Geometry: final body of the model. Coordinates: model frame, mm. A direction names the side the tool comes from. Coordinates: 2 decimals unless noted, no trailing zeros. Order: outer loops, then holes, each group sorted by start corner. A loop starts at its lowest first (then second) coordinate and runs counter-clockwise, first axis right, second up. Notation, with made-up numbers: (54, -20) - (72, -20) arc R12 cw to (72, -9) - close; hole circle Ø10 at (-21, 9). An arc over 180 degrees is marked (long way). Use one line per item in the form item = value. Start each with the question number.
```python
from build123d import *

# Parameters (mm, degrees)
SKETCH1_R               = 38.1
BOSS_EXTRUDE1_DEPTH     = 12.7
SKETCH2_W               = 30.48
SKETCH2_H               = 50.8
BOSS_EXTRUDE2_DEPTH     = 10.16
SKETCH3_W               = 25.4
SKETCH3_H               = 45.72
CUT_EXTRUDE1_DEPTH      = 10.16
BOSS_EXTRUDE3_DEPTH     = 127
SKETCH5_R               = 1.27
CUT_EXTRUDE2_DEPTH      = 5.08
SKETCH6_R               = 5.08
CUT_EXTRUDE3_DEPTH      = 5.08
SKETCH7_R               = 1.905
CUT_EXTRUDE4_DEPTH      = 57.658
CUT_EXTRUDE4_DEPTH_BACK = 54.61


with BuildPart() as part:
    # Sketch1 → Boss-Extrude1 (new body)
    with BuildSketch(Plane(origin=(0, 0, 0), x_dir=(1, 0, 0), z_dir=(0, 1, 0))):
        with Locations(Location((0, 0, 0), (0, 0, 270))):
            Circle(SKETCH1_R)
    extrude(amount=BOSS_EXTRUDE1_DEPTH)

    # Sketch2 → Boss-Extrude2 (add)
    with BuildSketch(Plane(origin=(0, 12.7, 0), x_dir=(1, 0, 0), z_dir=(0, 1, 0))):
        Rectangle(SKETCH2_W, SKETCH2_H)
    extrude(amount=BOSS_EXTRUDE2_DEPTH)

    # Sketch3 → Cut-Extrude1 (cut)
    with BuildSketch(Plane(origin=(0, 22.86, 0), x_dir=(1, 0, 0), z_dir=(0, 1, 0))):
        Rectangle(SKETCH3_W, SKETCH3_H)
    extrude(amount=-CUT_EXTRUDE1_DEPTH, mode=Mode.SUBTRACT)

    # Sketch4 → Boss-Extrude3 (add)
    with BuildSketch(Plane(origin=(0, 12.7, 0), x_dir=(1, 0, 0), z_dir=(0, 1, 0))):
        with BuildLine():
            Line((12.680636812, 25.4), (12.680636812, 35.927864535))
            ThreePointArc((12.680636812, 35.927864535), (38.1, 0), (12.680636812, -35.927864535))
            Line((12.680636812, -35.927864535), (12.680636812, 25.4))
        make_face()
    extrude(amount=BOSS_EXTRUDE3_DEPTH)

    # Sketch5 → Cut-Extrude2 (cut)
    with BuildSketch(Plane.ZY.offset(-12.680636812)):
        with Locations((-25.818357005, 129.781486407)):
            Circle(SKETCH5_R)
        with Locations((24.467398365, 129.781486407)):
            Circle(SKETCH5_R)
        with Locations((-25.818357005, 40.877093478)):
            Circle(SKETCH5_R)
        with Locations((24.467398365, 40.877093478)):
            Circle(SKETCH5_R)
    extrude(amount=-CUT_EXTRUDE2_DEPTH, mode=Mode.SUBTRACT)

    # Sketch6 → Cut-Extrude3 (cut)
    with BuildSketch(Plane(origin=(0, 139.7, 0), x_dir=(1, 0, 0), z_dir=(0, 1, 0))):
        with Locations(Location((25.4, 0, 0), (0, 0, 270))):
            Circle(SKETCH6_R)
    extrude(amount=-CUT_EXTRUDE3_DEPTH, mode=Mode.SUBTRACT)

    # Sketch7 → Cut-Extrude4 (cut, two sides)
    with BuildSketch(Plane(origin=(0, 0, 0), x_dir=(0, 0, -1), z_dir=(1, 0, 0))) as cut_extrude4_sk:
        with Locations(Location((0, 6.35, 0), (0, 0, 180))):
            Circle(SKETCH7_R)
    extrude(amount=CUT_EXTRUDE4_DEPTH, mode=Mode.SUBTRACT)
    extrude(cut_extrude4_sk.sketch, amount=-CUT_EXTRUDE4_DEPTH_BACK, mode=Mode.SUBTRACT)


solid = part.part
```
(1) Cut plane C-C on y = 6.35. Return the cut outline in (x, z) (3 decimals), plus the area to 3 significant figures.
(2) Draft query along X for faces 4 (the flat face through (-15.24, 18, 0)), 5 (the flat face through (0, 12.7, 0)), 6 (the flat face through (0, 18, -22.86)), 7 (the flat face through (20, 139.7, -1)). Return one class per face: released by +X, released by -X, zero draft, split by the parting line, or undercut.
(3) Cut plane B-B on x = -24. Return the cut outline in (y, z) (3 decimals), plus the area to 3 significant figures.
(4) Cut plane A-A on z = 0. Return the cut outline in (x, y) (3 decimals), plus the area to 3 significant figures.
(5) Material intervals for L1, parallel to Z at x = 7.5, y = 13; L2, parallel to Y at x = -13.5, z = 0 (3 decimals); L3, parallel to Y at x = -9, z = -33, sorted ascending. Write a range as from..to.
(6) Cut plane D-D on y = 83.5. Return the cut outline in (x, z), plus the area to 3 significant figures.
(7) Set-up query: faces 1 (the flat face through (-1, 18, -25.4)), 2 (the flat face through (25, 134.62, 0)), 3 (the flat face through (-1, 18, 25.4)). Return all of +Z, -Z, +X, -X, +Y, -Y with unobstructed straight access to the full face (end or side cutting, diameter ignored); none if empty.
(8) Contact query for flat-ended pins moving along their axis: pin 1 Ø0.8 at (y, z) = (41.5, -25.5) entering from -X; pin 2 Ø12 at (y, z) = (20.5, -4.5) entering from +X; pin 3 Ø1.5 at (y, z) = (40.88, -25.82) entering from +X. Output: stop coordinate, or through.
Check sheet entries:
q1.outline = (-38.052, -1.905) arc R38.1 ccw to (38.052, -1.905) - close; (-38.052, 1.905) - (38.052, 1.905) arc R38.1 ccw to start
q1.area = 4,270 mm^2
q2.face_4 = released by -X
q2.face_5 = undercut
q2.face_6 = undercut
q2.face_7 = zero draft
q3.outline = (0, -29.591) - (12.7, -29.591) - (12.7, 29.591) - (0, 29.591) - close; hole circle Ø3.81 at (6.35, 0)
q3.area = 740 mm^2
q4.outline = (-38.1, 0) - (38.1, 0) - (38.1, 4.445) - (-38.1, 4.445) - close; (-38.1, 8.255) - (38.1, 8.255) - (38.1, 139.7) - (30.48, 139.7) - (30.48, 134.62) - (20.32, 134.62) - (20.32, 139.7) - (12.681, 139.7) - (12.681, 12.7) - (-12.7, 12.7) - (-12.7, 22.86) - (-15.24, 22.86) - (-15.24, 12.7) - (-38.1, 12.7) - close
q4.area = 3,880 mm^2
q5.L1 = -25.4..-22.86, 22.86..25.4
q5.L2 = 0..4.445, 8.255..22.86
q5.L3 = 0..12.7
q6.outline = (12.68, -35.93) arc R38.1 ccw to (12.68, 35.93) - close
q6.area = 1,330 mm^2
q7.face_1 = -Z, -X, +Y
q7.face_2 = +Y
q7.face_3 = +Z, -X, +Y
q8.pin_1 = 17.76
q8.pin_2 = 38.1
q8.pin_3 = 28.69
